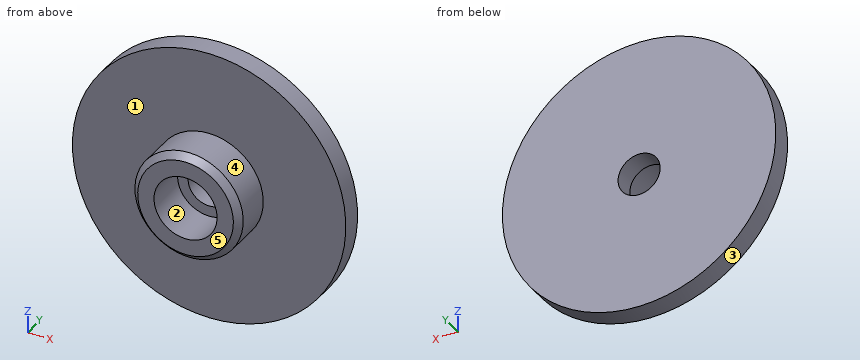
Solid Edge part; units mm, degrees
sketch "Sketch1" plane through (0, 0, 0) normal (1, 0, 0) x (0, 1, 0)
  line L0 (0, 65) -> (0, 25.75)
  line L1 (0, 25.75) -> (-20, 25.75)
  line L2 (-20, 25.75) -> (-20, 0)
  line L3 (-20, 0) -> (10, 0)
  line L4 (10, 0) -> (10, 65)
  line L5 (10, 65) -> (0, 65)
revolve "RevolvedProtrusion1" add sketch "Sketch1" angle 360 about axis through (0, -20, 0) along (0, 1, 0)
hole "Agujero_1" at (0, -20, 0) direction (0, 1, 0) diameter 20 end up to next counterbore diameter 30 counterbore depth 20
chamfer "Chaflán_1" distance 3 angle 45 1 edges at (0, -20, 25.75)
properties material "Acero ASTM A36"
Geometry: final body of the model. Coordinates: model frame, mm. Face numbers are marked on the shaded views. A direction names the side the tool comes from. Give positions to 0.01 mm unless a question says otherwise; leave off trailing zeros. Write each loop counter-clockwise with the first axis right and the second up, starting at its lowest first coordinate (ties: lowest second). Pieces come first, ordered by that corner, then holes. Notation, with made-up numbers: (50.5, 0) - (89.5, 0) arc R27 cw to (89.5, 23) - close; hole circle Ø2 at (52.25, 89.25). An arc over 180 degrees is marked (long way). Return JSON: item names as keys, results as strings. Group by question number.
1) First-contact query: P1, Ø6, axis at x = 14, y = 3.5, coming from the -Z side; P2, Ø2, axis at x = 27.5, z = -13.5, coming from the -Y side; P3, Ø6, axis at x = -34, y = 3, coming from the +Z side. Flat tips, straight axial feed; report the tip coordinate or a pass-through.
2) Section C-C on y = 7.25. Return the cut outline in (x, z).
3) Set-up query: the marked faces 4 and 5. Return all of +Z, -Z, +X, -X, +Y, -Y with unobstructed straight access to the full face (end or side cutting, diameter ignored); none if empty.
4) Section B-B on z = 0. Return the cut outline in (x, y), plus the area to 3 significant figures.
5) Section A-A on x = 0. Return the cut outline in (y, z).
6) Mould query, pull axis Z, two halves, no side actions, for the marked faces 1, 2 and 3. Classes: released by +Z, released by -Z, zero draft, split by the parting line, or undercut.
7) Section D-D on y = -10.75. Return the cut outline in (x, z).
8) Line query: line 1 (X direction, y = -12.75, z = 0); line 2 (X direction, y = 7, z = 0); line 3 (Y direction, x = 52, z = 35). Output: solid intervals per line, ascending.
Filled in:
{
 "1": {"P1": "stops at z = -64.06", "P2": "stops at y = 0", "P3": "stops at z = 57.13"},
 "2": {"outline": "circle Ø130 at (0, 0); hole circle Ø20 at (0, 0)"},
 "3": {"face 4": "-Y", "face 5": "+Z, -Z, +X, -X, -Y"},
 "4": {"outline": "(-65, 0) - (-25.75, 0) - (-25.75, -17) - (-22.75, -20) - (-15, -20) - (-15, 0) - (-10, 0) - (-10, 10) - (-65, 10) - close; (10, 0) - (15, 0) - (15, -20) - (22.75, -20) - (25.75, -17) - (25.75, 0) - (65, 0) - (65, 10) - (10, 10) - close", "area": "1,520 mm^2"},
 "5": {"outline": "(-20, -22.75) - (-17, -25.75) - (0, -25.75) - (0, -65) - (10, -65) - (10, -10) - (0, -10) - (0, -15) - (-20, -15) - close; (-20, 15) - (0, 15) - (0, 10) - (10, 10) - (10, 65) - (0, 65) - (0, 25.75) - (-17, 25.75) - (-20, 22.75) - close"},
 "6": {"face 1": "zero draft", "face 2": "undercut", "face 3": "split by the parting line"},
 "7": {"outline": "circle Ø51.5 at (0, 0); hole circle Ø30 at (0, 0)"},
 "8": {"line 1": "x = -25.75 to -15, 15 to 25.75", "line 2": "x = -65 to -10, 10 to 65", "line 3": "y = 0 to 10"}
}
